```python
from build123d import *
from build123d.topology import SkipClean

# Parameters (mm, degrees)
SKETCH1_W             = 65
SKETCH1_H             = 9
BOSS_EXTRUDE1_DEPTH   = 45
BOSS_EXTRUDE1_2_DEPTH = 45
CUT_EXTRUDE5_DEPTH    = 34
CUT_EXTRUDE6_DEPTH    = 34
SKETCH3_R             = 3
CUT_EXTRUDE7_DEPTH    = 2.45
SKETCH4_R             = 3
CUT_EXTRUDE8_DEPTH    = 2.45
SKETCH5_W             = 65
SKETCH5_H             = 29
BOSS_EXTRUDE2_DEPTH   = 2.45
SKETCH6_W             = 7
SKETCH6_H             = 6.853915881
SKETCH6_R             = 0.75
BOSS_EXTRUDE3_DEPTH   = 3.35
CUT_EXTRUDE9_DEPTH    = 3.35
BOSS_EXTRUDE4_DEPTH   = 2
SKETCH9_W             = 6.962412957
SKETCH9_H             = 29
BOSS_EXTRUDE5_DEPTH   = 73
SKETCH10_R            = 3
CUT_EXTRUDE10_DEPTH   = 2.5
CUT_EXTRUDE11_START   = -2.5
SKETCH11_R            = 3
CUT_EXTRUDE11_DEPTH   = 2.5
SKETCH12_R            = 1
CUT_EXTRUDE12_DEPTH   = 32.5
SKETCH13_W            = 25.743716973
SKETCH13_H            = 29
BOSS_EXTRUDE6_DEPTH   = 20.5
SKETCH14_W            = 16.2
SKETCH14_H            = 32.7
CUT_EXTRUDE13_DEPTH   = 17.5
SKETCH16_W            = 16.2
SKETCH16_H            = 3.197897976
SKETCH16_H_2          = 3.137509592
BOSS_EXTRUDE7_DEPTH   = 17.5
SKETCH17_W            = 2.5
SKETCH17_H            = 3.197897976
SKETCH17_H_2          = 3.137509592
CUT_EXTRUDE14_DEPTH   = 17.5
SKETCH19_R            = 1
CUT_EXTRUDE15_DEPTH   = 10
SKETCH20_R            = 3.481206478
BOSS_EXTRUDE8_DEPTH   = 6
CUT_EXTRUDE17_DEPTH   = 66


# Read off the part's stored shape, not the designer's step: Boss-Extrude4
with BuildPart() as part:
    # Sketch1 → Boss-Extrude1 (new body)
    with BuildSketch(Plane.XY):
        with Locations((32.5, 15.5)):
            Rectangle(SKETCH1_W, SKETCH1_H)
    extrude(amount=BOSS_EXTRUDE1_DEPTH)


with BuildPart() as body_2:
    # Sketch1 → Boss-Extrude1 2 (new body)
    with BuildSketch(Plane.XY):
        with Locations((32.5, 35.5)):
            Rectangle(SKETCH1_W, SKETCH1_H)
    extrude(amount=BOSS_EXTRUDE1_2_DEPTH)


with BuildPart() as cut_extrude5_tool:
    # Sketch2 → Cut-Extrude5 (new body)
    with BuildSketch(Plane.XZ.offset(-10)):
        with BuildLine():
            ThreePointArc((45.80925577, 8.081639583), (40.285389963, 2.178623197), (32.5, 0))
            Line((32.5, 0), (65, 0))
            Line((65, 0), (65, 45))
            Line((65, 45), (45.80925577, 8.081639583))
        make_face()
        with BuildLine():
            Line((32.5, 16), (32.5, 14))
            ThreePointArc((32.5, 14), (33.207106781, 14.292893219), (33.5, 15))
            ThreePointArc((33.5, 15), (33.207106781, 15.707106781), (32.5, 16))
        make_face()
        with BuildLine():
            ThreePointArc((32.5, 16), (31.5, 15), (32.5, 14))
            Line((32.5, 14), (32.5, 16))
        make_face()
    extrude(amount=-CUT_EXTRUDE5_DEPTH)


with BuildPart() as part_1:
    add(part.part)

    # Cut-Extrude5: cut by cut_extrude5_tool
    add(cut_extrude5_tool.part, mode=Mode.SUBTRACT)


with BuildPart() as body_2_1:
    add(body_2.part)

    # Cut-Extrude5: cut by cut_extrude5_tool
    add(cut_extrude5_tool.part, mode=Mode.SUBTRACT)


with BuildPart() as cut_extrude6_tool:
    # Sketch2_6 → Cut-Extrude6 (new body)
    with BuildSketch(Plane.XZ.offset(-10)):
        with BuildLine():
            Line((19.19074423, 8.081639583), (0, 45))
            Line((0, 45), (0, 0))
            Line((0, 0), (32.5, 0))
            ThreePointArc((32.5, 0), (24.714610037, 2.178623197), (19.19074423, 8.081639583))
        make_face()
    extrude(amount=-CUT_EXTRUDE6_DEPTH)


with BuildPart() as part_2:
    add(part_1.part)

    # Cut-Extrude6: cut by cut_extrude6_tool
    add(cut_extrude6_tool.part, mode=Mode.SUBTRACT)

    # Sketch4 → Cut-Extrude8 (cut)
    with BuildSketch(Plane(origin=(0, 20, 0), x_dir=(1, 0, 0), z_dir=(0, 1, 0))):
        with Locations(Location((32.5, -15, 0), (0, 0, 270))):
            Circle(SKETCH4_R)
    extrude(amount=-CUT_EXTRUDE8_DEPTH, mode=Mode.SUBTRACT)



with BuildPart() as body_2_2:
    add(body_2_1.part)

    # Cut-Extrude6: cut by cut_extrude6_tool
    add(cut_extrude6_tool.part, mode=Mode.SUBTRACT)

    # Sketch3 → Cut-Extrude7 (cut)
    with BuildSketch(Plane(origin=(0, 40, 0), x_dir=(1, 0, 0), z_dir=(0, 1, 0))):
        with Locations(Location((32.5, -15, 0), (0, 0, 270))):
            Circle(SKETCH3_R)
    extrude(amount=-CUT_EXTRUDE7_DEPTH, mode=Mode.SUBTRACT)


with BuildPart() as part_3:
    add(part_2.part)

    add(body_2_2.part)  # Boss-Extrude2 merges body 2
    # Sketch5 → Boss-Extrude2 (add)
    with BuildSketch(Plane.XY.offset(45)):
        with Locations((32.5, 25.5)):
            Rectangle(SKETCH5_W, SKETCH5_H)
    extrude(amount=BOSS_EXTRUDE2_DEPTH)

    # Sketch6 → Boss-Extrude3 (add)
    with BuildSketch(Plane.XZ.offset(-11)):
        with Locations((32.5, 30.126957941)):
            Rectangle(SKETCH6_W, SKETCH6_H)
        with Locations(Location((32.5, 28.3, 0), (0, 0, 270))):
            Circle(SKETCH6_R, mode=Mode.SUBTRACT)
    extrude(amount=BOSS_EXTRUDE3_DEPTH)

    # Sketch7 → Cut-Extrude9 (cut)
    with BuildSketch(Plane.XZ.offset(-7.65)):
        Polygon((29, 29.7), (29, 26.7), (31, 26.7), align=None)
        Polygon((34, 26.7), (36, 29.7), (36, 26.7), align=None)
    extrude(amount=-CUT_EXTRUDE9_DEPTH, mode=Mode.SUBTRACT)

    # Boss-Extrude4 outline → Boss-Extrude4 (add)
    with BuildSketch(Plane.XZ.offset(-7.65)):
        with BuildLine():
            Line((36, 29.7), (36, 33.553915881))
            Line((36, 33.553915881), (29, 33.553915881))
            Line((29, 33.553915881), (29, 29.7))
            Line((29, 29.7), (30.278889745, 27.781665383))
            Line((30.278889745, 27.781665383), (30.454857608, 30.333257))
            ThreePointArc((30.454857608, 30.333257), (32.5, 32.242215881), (34.545142392, 30.333257))
            Line((34.545142392, 30.333257), (34.721110255, 27.781665383))
            Line((34.721110255, 27.781665383), (36, 29.7))
        make_face()
    extrude(amount=BOSS_EXTRUDE4_DEPTH)

    # Sketch9 → Boss-Extrude5 (add)
    with BuildSketch(Plane.XY.offset(47.45)):
        with Locations((61.518793522, 25.5)):
            Rectangle(SKETCH9_W, SKETCH9_H)
    extrude(amount=BOSS_EXTRUDE5_DEPTH)

    # Sketch10 → Cut-Extrude10 (cut)
    with BuildSketch(Plane.XZ.offset(-11)):
        with Locations(Location((45.037587043, 42.45, 0), (0, 0, 270))):
            Circle(SKETCH10_R)
    extrude(amount=-CUT_EXTRUDE10_DEPTH, mode=Mode.SUBTRACT)

    # Sketch11 → Cut-Extrude11 (cut)
    with BuildSketch(Plane(origin=(0, 40, 0), x_dir=(1, 0, 0), z_dir=(0, 1, 0)).offset(CUT_EXTRUDE11_START)):
        with Locations(Location((45.037587043, -42.45, 0), (0, 0, 90))):
            Circle(SKETCH11_R)
    extrude(amount=CUT_EXTRUDE11_DEPTH, mode=Mode.SUBTRACT)

    # Sketch12 → Cut-Extrude12 (cut)
    with BuildSketch(Plane(origin=(0, 37.5, 0), x_dir=(1, 0, 0), z_dir=(0, 1, 0))):
        with Locations(Location((45.037587043, -42.45, 0), (0, 0, 180))):
            Circle(SKETCH12_R)
    extrude(amount=-CUT_EXTRUDE12_DEPTH, mode=Mode.SUBTRACT)

    # Sketch13 → Boss-Extrude6 (add)
    with BuildSketch(Plane.XY.offset(47.45)):
        with Locations((12.871858487, 25.5)):
            Rectangle(SKETCH13_W, SKETCH13_H)
    extrude(amount=BOSS_EXTRUDE6_DEPTH)

    # Sketch14 → Cut-Extrude13 (cut)
    with BuildSketch(Plane(origin=(25.743716973, 0, 0), x_dir=(0, 0, -1), z_dir=(1, 0, 0))):
        with Locations((-55.55, 25.5)):
            Rectangle(SKETCH14_W, SKETCH14_H)
    extrude(amount=-CUT_EXTRUDE13_DEPTH, mode=Mode.SUBTRACT)

    # Sketch16 → Boss-Extrude7 (add)
    with BuildSketch(Plane(origin=(8.243716973, 0, 0), x_dir=(0, 0, -1), z_dir=(1, 0, 0))):
        with Locations((-55.55, 12.598948988)):
            Rectangle(SKETCH16_W, SKETCH16_H)
        with Locations((-55.55, 38.431245204)):
            Rectangle(SKETCH16_W, SKETCH16_H_2)
    extrude(amount=BOSS_EXTRUDE7_DEPTH)

    # Sketch17 → Cut-Extrude14 (cut)
    with BuildSketch(Plane(origin=(25.743716973, 0, 0), x_dir=(0, 0, -1), z_dir=(1, 0, 0))):
        Polygon((-67.95, 36.862490408), (-67.95, 14.197897976), (-66.15, 14.197897976), (-63.65, 14.197897976), (-63.65, 36.862490408), (-66.15, 36.862490408), align=None)
        with Locations((-64.9, 12.598948988)):
            Rectangle(SKETCH17_W, SKETCH17_H)
        with Locations((-64.9, 38.431245204)):
            Rectangle(SKETCH17_W, SKETCH17_H_2)
    extrude(amount=-CUT_EXTRUDE14_DEPTH, mode=Mode.SUBTRACT)

    # Sketch19 → Cut-Extrude15 (cut)
    with BuildSketch(Plane.XY.offset(67.95)):
        with Locations((21.843716973, 12.598948988)):
            Circle(SKETCH19_R)
        with Locations((21.843716973, 38.431245204)):
            Circle(SKETCH19_R)
    extrude(amount=-CUT_EXTRUDE15_DEPTH, mode=Mode.SUBTRACT)

    # Sketch20 → Boss-Extrude8 (add)
    with BuildSketch(Plane.XZ.offset(-11)):
        with Locations(Location((61.518793522, 65.411058123, 0), (0, 0, 180))):
            Circle(SKETCH20_R)
    extrude(amount=BOSS_EXTRUDE8_DEPTH)

    # Sketch22 → Cut-Extrude17 (cut)
    with SkipClean():  # the faces are left unmerged after this step: merging them gives an invalid solid
        with BuildSketch(Plane.XY.offset(120.45)):
            Polygon((65, 7.755866492), (65, 11), (64, 7.755866492), align=None)
            Polygon((65, 5), (65, 7.755866492), (64, 7.755866492), align=None)
        extrude(amount=-CUT_EXTRUDE17_DEPTH, mode=Mode.SUBTRACT)


solid = part_3.part
```
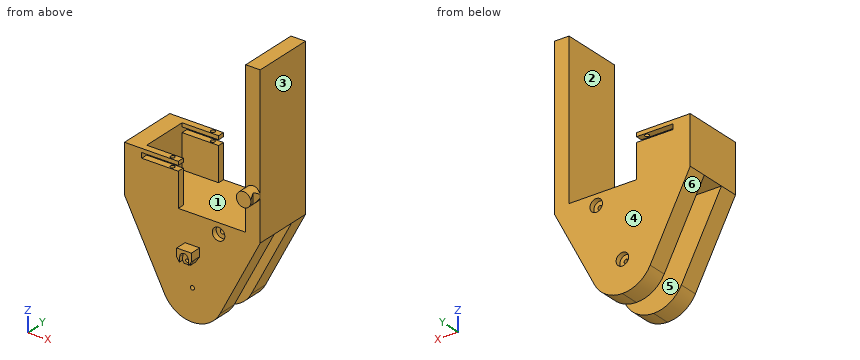
Work out the finished part from the listing and answer in its coordinate system (mm). Face numbers are marked on the shaded views. A direction names the side the tool comes from. Coordinates: 2 decimals unless noted, no trailing zeros. Write each loop counter-clockwise with the first axis right and the second up, starting at its lowest first coordinate (ties: lowest second). Pieces come first, ordered by that corner, then holes. Notation, with made-up numbers: (45, 89.5) - (66, 89.5) arc R9 cw to (66, 94.5) - close; hole circle Ø5 at (-4, 9). An arc over 180 degrees is marked (long way). Answer as a JSON object with one key per item and string values.
Q1. Consider L1, parallel to Y at x = 19.5, z = 54.5; L2, parallel to Z at x = 32.5, y = 8.8; L3, parallel to X at y = 28, z = 66. Determine where each line is inside the solid, lowest interval first. Write a range as from..to.
Results list:
{"L1": "y = 11..14.2, 36.86..40", "L2": "z = 26.7..27.55, 29.05..33.55", "L3": "x = 0..8.24, 58.04..65"}
Q2. Find section A-A (y = 9). Write down the section's boundary in (x, z), plus the area to 3 significant figures.
Results list:
{"outline": "(29, 29.7) - (31, 26.7) - (34, 26.7) - (36, 29.7) - (36, 33.55) - (29, 33.55) - close; (64.38, 63.43) - (64.38, 67.39) arc R3.48 ccw (long way) to start; hole circle Ø1.5 at (32.5, 28.3)", "area": "76.6 mm^2"}
Q3. Find section B-B (z = 99). Write down the section's boundary in (x, y).
Results list:
{"outline": "(58.04, 11) - (65, 11) - (65, 40) - (58.04, 40) - close"}
Q4. For a pull along Y with two mould halves and no side action, classify the marked faces 4, 5 and 6 as pulls with the +Y half, pulls with the -Y half, needs draft (parallel to the pull), parting line crosses it, or undercut.
Results list:
{"face 4": "pulls with the +Y half", "face 5": "undercut", "face 6": "needs draft"}
Q5. Given pin 1 Ø6 at (x, z) = (55, 38) entering from -Y; pin 2 Ø3 at (x, z) = (45, 41.5) entering from +Y; pin 3 Ø1.2 at (y, z) = (9, 31.5) entering from +X, each flat-ended and moving along its own axis, determine where each tip first touches the part or whether it passes through.
Results list:
{"pin 1": "stops at y = 11", "pin 2": "stops at y = 37.5", "pin 3": "stops at x = 36"}
Q6. Find section D-D (x = 7). Write down the section's boundary in (y, z), plus the area to 3 significant figures.
Results list:
{"outline": "(11, 31.53) - (20, 31.53) - (20, 45) - (31, 45) - (31, 31.53) - (40, 31.53) - (40, 67.95) - (11, 67.95) - close", "area": "908 mm^2"}
Q7. Find section C-C (x = 56). Write down the section's boundary in (y, z), plus the area to 3 significant figures.
Results list:
{"outline": "(11, 27.69) - (20, 27.69) - (20, 45) - (31, 45) - (31, 27.69) - (40, 27.69) - (40, 47.45) - (11, 47.45) - close", "area": "383 mm^2"}
Q8. Which of the six approach directions +Z, -Z, +X, -X, +Y, -Y give full straight-line access (tool end or side, diameter ignored) to the marked faces 1, 2 and 3?
Results list:
{"face 1": "+Z", "face 2": "+Z, +Y, -Y", "face 3": "+Z, -Z, +X, +Y, -Y"}
